Source: CAD feature listing. Evaluate the final solid. Frame: model axes, mm. A direction names the side the tool comes from. Round coordinates to 2 decimals unless told otherwise and drop trailing zeros. Loops run counter-clockwise (first coordinate to the right, second up) from the corner with the lowest first, then second, coordinate; pieces in that order, holes last.
Item 1: Access query for faces 1 (the flat face through (288.006, 5.67, -147.258)), 2 (the flat face through (244, 0, -223)). Directions: +Z, -Z, +X, -X, +Y, -Y. A direction counts if a zero-diameter tool reaches every point of the face in a straight line with its end or side. Return the directions, or none.
Item 2: Section query A-A on y = 9. Return loops of the section in (x, z), then the cut area to 3 significant figures.
Item 3: Section query D-D on x = 90. Return loops of the section in (y, z).
Item 4: First-contact query: P1, Ø2, axis at y = 8.5, z = -207, coming from the +X side; P2, Ø3.5, axis at x = 586, y = 4, coming from the +Z side; P3, Ø6, axis at y = 7, z = -181.5, coming from the -X side. Flat tips, straight axial feed; report the tip coordinate or a pass-through.
Item 5: Section query C-C on x = -175. Return loops of the section in (y, z) (3 decimals), then the cut area to 3 significant figures.
Item 6: Section query B-B on z = -119. Return loops of the section in (x, y).
Item 7: Ray query, L1, parallel to X at y = 6.5, z = -273.5; L2, parallel to X at y = 10.25, z = -254; L3, parallel to Z at x = 149.5, y = 5. Return the intervals inside material, ascending.
Item 8: Pull-direction query (Z, two-part tool) for faces 3 (the flat face through (310.89, 5.67, -154.4)), 4 (the flat face through (-222.18, 5.67, -152.26)), 5 (the flat face through (244, 11.5, -223)); classes: released by +Z, released by -Z, zero draft, split by the parting line, or undercut.
```python
from build123d import *

# Parameters (mm, degrees)
BOSS_EXTRUDE2_DEPTH = 11.5
CUT_EXTRUDE3_REACH  = 892.817


with BuildPart() as part:
    # Sketch1 → Boss-Extrude2 (new body)
    with BuildSketch(Plane(origin=(0, 0, 0), x_dir=(1, 0, 0), z_dir=(0, 1, 0))):
        Polygon((-434.5, 311.5), (-3.833333333, -11.5), (403.833333333, -11.5), (834.5, 311.5), align=None)
    extrude(amount=BOSS_EXTRUDE2_DEPTH)

    # Sketch1_8 → Cut-Extrude3 (cut, up to next)
    with BuildSketch(Plane(origin=(0, 0, 0), x_dir=(1, 0, 0), z_dir=(0, 1, 0)), mode=Mode.PRIVATE) as cut_extrude3_sk1:
        Polygon((200, 279.268080166), (378.512053444, 11.5), (21.487946556, 11.5), align=None)
    cut_extrude3_tool1 = extrude(cut_extrude3_sk1.sketch, amount=CUT_EXTRUDE3_REACH, mode=Mode.PRIVATE) & part.part
    # Sketch1_8 → Cut-Extrude3 (cut, up to next)
    with BuildSketch(Plane(origin=(0, 0, 0), x_dir=(1, 0, 0), z_dir=(0, 1, 0)), mode=Mode.PRIVATE) as cut_extrude3_sk2:
        Polygon((178.512053444, 288.5), (-2.825297704, 16.493973278), (-365.5, 288.5), align=None)
    cut_extrude3_tool2 = extrude(cut_extrude3_sk2.sketch, amount=CUT_EXTRUDE3_REACH, mode=Mode.PRIVATE) & part.part
    # Sketch1_8 → Cut-Extrude3 (cut, up to next)
    with BuildSketch(Plane(origin=(0, 0, 0), x_dir=(1, 0, 0), z_dir=(0, 1, 0)), mode=Mode.PRIVATE) as cut_extrude3_sk3:
        Polygon((765.5, 288.5), (221.487946556, 288.5), (402.825297704, 16.493973278), align=None)
    cut_extrude3_tool3 = extrude(cut_extrude3_sk3.sketch, amount=CUT_EXTRUDE3_REACH, mode=Mode.PRIVATE) & part.part
    add(cut_extrude3_tool1.solids().sort_by_distance((200, 0, -100.756027))[0], mode=Mode.SUBTRACT)
    add(cut_extrude3_tool2.solids().sort_by_distance((-63.271081, 0, -197.831324))[0], mode=Mode.SUBTRACT)
    add(cut_extrude3_tool3.solids().sort_by_distance((463.271081, 0, -197.831324))[0], mode=Mode.SUBTRACT)


solid = part.part
```
Data:
1. face 1: +Y, -Y
1. face 2: +Z, -Z, +X, -X, -Y
2. outline: (-434.5, -311.5) - (834.5, -311.5) - (403.83, 11.5) - (-3.83, 11.5) - close; hole (-365.5, -288.5) - (178.51, -288.5) - (-2.83, -16.49) - close; hole (21.49, -11.5) - (200, -279.27) - (378.51, -11.5) - close; hole (221.49, -288.5) - (765.5, -288.5) - (402.83, -16.49) - close
2. area: 75,000 mm2
3. outline: (0, -311.5) - (11.5, -311.5) - (11.5, -288.5) - (0, -288.5) - close; (0, -155.73) - (11.5, -155.73) - (11.5, -114.27) - (0, -114.27) - close; (0, -11.5) - (11.5, -11.5) - (11.5, 11.5) - (0, 11.5) - close
4. P1: stops at x = 696.5
4. P2: stops at z = -123.81
4. P3: stops at x = -265.17
5. outline: (0, -311.5) - (11.5, -311.5) - (11.5, -288.5) - (0, -288.5) - close; (0, -145.625) - (11.5, -145.625) - (11.5, -116.875) - (0, -116.875) - close
5. area: 595 mm2
6. outline: (-177.83, 0) - (-139.5, 0) - (-139.5, 11.5) - (-177.83, 11.5) - close; (65.51, 0) - (93.15, 0) - (93.15, 11.5) - (65.51, 11.5) - close; (306.85, 0) - (334.49, 0) - (334.49, 11.5) - (306.85, 11.5) - close; (539.5, 0) - (577.83, 0) - (577.83, 11.5) - (539.5, 11.5) - close
7. L1: x = -383.83 to -345.5, 168.51 to 196.15, 203.85 to 231.49, 745.5 to 783.83
7. L2: x = -357.83 to -319.5, 155.51 to 183.15, 216.85 to 244.49, 719.5 to 757.83
7. L3: z = -311.5 to -288.5, -244.98 to -203.52, -11.5 to 11.5
8. face 3: undercut
8. face 4: released by +Z
8. face 5: zero draft
